Geometry check sheet. Reference: the model listing, model coordinates, mm. Coordinates: 2 decimals unless noted, no trailing zeros. One line per question, with ' | ' between items.
```python
from build123d import *

# Parameters (mm, degrees)
F0_R     = 3.5
F1_DEPTH = 50.8


with BuildPart() as f1:
    # F0 (on Top) → F1 (new body)
    with BuildSketch(Plane.XY):
        with BuildLine():
            add(Edge.make_bspline(
                [(-60.727015, 0), (-6.678293, 15.829317), (18.438485, 17.843956), (46.355639, 18.419569)],
                knots=[0, 0, 0, 0, 108.655305, 108.655305, 108.655305, 108.655305], degree=3))
            Line((-60.727015, 0), (73.772119, 0))
            add(Edge.make_bspline(
                [(46.355639, 18.419569), (61.652482, 19.117288), (71.317069, 6.619532), (73.772119, 0)],
                knots=[0, 0, 0, 0, 33.029441, 33.029441, 33.029441, 33.029441], degree=3))
        make_face()
        with Locations((-7.635186, 5.816073)):
            Circle(F0_R, mode=Mode.SUBTRACT)
        with Locations((48.322952, 6.087539)):
            Circle(F0_R, mode=Mode.SUBTRACT)
    extrude(amount=F1_DEPTH)


solid = f1.part
```
(1) Material ranges on line 1 (Y direction, x = 29, z = 44.5); line 2 (Y direction, x = -1, z = 23), recorded low to high.
Answers below:
line 1: y = 0 to 17.76 | line 2: y = 0 to 14.35
(2) Depth check by flat-ended pin: P1, Ø9, axis at x = -7.64, y = 5.82, coming from the -Z side; P2, Ø1.5, axis at x = -46, z = 37, coming from the +Y side; P3, Ø3, axis at x = 27, z = 9, coming from the +Y side. Enter the tip coordinate at first touch or a pass-through.
Answers below:
P1: stops at z = 0 | P2: stops at y = 4.37 | P3: stops at y = 17.73
(3) Draft check along X on faces 1 (the face through (6, 0, 25)), 2 (the face through (44.826, 6.241, 25.044)). Enter one of: pulls with the +X half, pulls with the -X half, needs draft (parallel to the pull), parting line crosses it, or undercut.
Answers below:
face 1: needs draft | face 2: undercut
(4) Cross-section at A-A (y = 7.5). Count the separate pieces of the cut face and the enclosed holes in it, plus the area to 3 significant figures.
Answers below:
separate pieces: 3 | enclosed holes: 0 | area: 4,570 mm²
